from build123d import *

# Parameters (mm, degrees)
SKETCH1_W               = 44
SKETCH1_H               = 95
BOSS_EXTRUDE1_DEPTH     = 25
SKETCH2_W               = 38
SKETCH2_H               = 89
CUT_EXTRUDE1_DEPTH      = 22
CHAMFER1_SIZE           = 10
FILLET1_R               = 2
FILLET2_R               = 5
SKETCH3_W               = 14
SKETCH3_H               = 10
BOSS_EXTRUDE2_DEPTH     = 7
SKETCH5_W               = 14
SKETCH5_H               = 10
BOSS_EXTRUDE3_DEPTH     = 7
FILLET3_R               = 3
CUT_EXTRUDE2_DEPTH      = 62.010245041
CUT_EXTRUDE2_DEPTH_BACK = 62.010245041
SKETCH7_W               = 3
SKETCH7_H               = 6
SKETCH8_R               = 3
CUT_EXTRUDE3_DEPTH      = 10


with BuildPart() as part:
    # Sketch1 → Boss-Extrude1 (new body)
    with BuildSketch(Plane(origin=(0, 0, 0), x_dir=(1, 0, 0), z_dir=(0, 1, 0))):
        Rectangle(SKETCH1_W, SKETCH1_H)
    extrude(amount=BOSS_EXTRUDE1_DEPTH)

    # Sketch2 → Cut-Extrude1 (cut)
    with BuildSketch(Plane(origin=(0, 25, 0), x_dir=(1, 0, 0), z_dir=(0, 1, 0))):
        Rectangle(SKETCH2_W, SKETCH2_H)
    extrude(amount=-CUT_EXTRUDE1_DEPTH, mode=Mode.SUBTRACT)

    # Chamfer1
    chamfer1_edges = [part.edges().sort_by_distance(p)[0] for p in [
        (-19, 3, 0),
        (0, 3, -44.5),
        (19, 3, 0),
        (0, 3, 44.5),
        (0, 0, 47.5),
        (-22, 0, 0),
        (0, 0, -47.5),
        (22, 0, 0),
    ]]
    chamfer(chamfer1_edges, length=CHAMFER1_SIZE)

    # Fillet1
    fillet1_edges = [part.edges().sort_by_distance(p)[0] for p in [
        (-19, 19, -44.5),
        (19, 19, -44.5),
        (19, 19, 44.5),
        (-19, 19, 44.5),
    ]]
    fillet(fillet1_edges, radius=FILLET1_R)

    # Fillet2
    fillet2_edges = [part.edges().sort_by_distance(p)[0] for p in [
        (22, 17.5, 47.5),
        (-22, 17.5, 47.5),
        (-22, 17.5, -47.5),
        (22, 17.5, -47.5),
    ]]
    fillet(fillet2_edges, radius=FILLET2_R)

    # Sketch3 → Boss-Extrude2 (add)
    with BuildSketch(Plane(origin=(22, 0, 0), x_dir=(0, 0, -1), z_dir=(1, 0, 0))):
        with Locations((-32.5, 20)):
            Rectangle(SKETCH3_W, SKETCH3_H)
        with Locations((32.5, 20)):
            Rectangle(SKETCH3_W, SKETCH3_H)
    extrude(amount=BOSS_EXTRUDE2_DEPTH)

    # Sketch5 → Boss-Extrude3 (add)
    with BuildSketch(Plane.ZY.offset(22)):
        with Locations((32.5, 20)):
            Rectangle(SKETCH5_W, SKETCH5_H)
        with Locations((-32.5, 20)):
            Rectangle(SKETCH5_W, SKETCH5_H)
    extrude(amount=BOSS_EXTRUDE3_DEPTH)

    # Fillet3
    fillet3_edges = [part.edges().sort_by_distance(p)[0] for p in [
        (22, 20, 39.5),
        (22, 15, 32.5),
        (25.5, 15, 39.5),
        (22, 20, 25.5),
        (25.5, 15, 25.5),
        (29, 20, 39.5),
        (29, 15, 32.5),
        (29, 20, 25.5),
        (22, 20, -25.5),
        (22, 15, -32.5),
        (25.5, 15, -25.5),
        (22, 20, -39.5),
        (25.5, 15, -39.5),
        (29, 20, -25.5),
        (29, 15, -32.5),
        (29, 20, -39.5),
        (-22, 20, 39.5),
        (-25.5, 15, 39.5),
        (-22, 20, 25.5),
        (-22, 15, 32.5),
        (-25.5, 15, 25.5),
        (-29, 20, 39.5),
        (-29, 20, 25.5),
        (-29, 15, 32.5),
        (-22, 15, -32.5),
        (-25.5, 15, -39.5),
        (-22, 20, -25.5),
        (-25.5, 15, -25.5),
        (-22, 20, -39.5),
        (-29, 15, -32.5),
        (-29, 20, -25.5),
        (-29, 20, -39.5),
    ]]
    fillet(fillet3_edges, radius=FILLET3_R - 0.0001)  # a hair under: the kernel refuses the full size

    # Sketch7 → Cut-Extrude2 (cut, two sides: drawn at the far end of the back side and taken through both)
    with BuildSketch(Plane(origin=(0, 25, 0), x_dir=(1, 0, 0), z_dir=(0, 1, 0)).offset(-CUT_EXTRUDE2_DEPTH_BACK)):
        with Locations((-23.5, 32.5)):
            Rectangle(SKETCH7_W, SKETCH7_H)
        with Locations((23.5, 32.5)):
            Rectangle(SKETCH7_W, SKETCH7_H)
        with Locations((23.5, -32.5)):
            Rectangle(SKETCH7_W, SKETCH7_H)
        with Locations((-23.5, -32.5)):
            Rectangle(SKETCH7_W, SKETCH7_H)
    extrude(amount=CUT_EXTRUDE2_DEPTH + CUT_EXTRUDE2_DEPTH_BACK, mode=Mode.SUBTRACT)

    # Sketch8 → Cut-Extrude3 (cut)
    with BuildSketch(Plane.XY.offset(47.5)):
        with Locations((7, 25)):
            Circle(SKETCH8_R)
        with Locations((-7, 25)):
            Circle(SKETCH8_R)
    extrude(amount=-CUT_EXTRUDE3_DEPTH, mode=Mode.SUBTRACT)


solid = part.part
For this review, take the finished solid that the model builds, in its own axes (mm). A direction names the side the tool comes from. Coordinates: 2 decimals unless noted, no trailing zeros. Order: outer loops, then holes, each group sorted by start corner. A loop starts at its lowest first (then second) coordinate and runs counter-clockwise, first axis right, second up. Notation, with made-up numbers: (-33, 21.25) - (-17, 21.25) arc R25 ccw to (-17, 45.25) - close; hole circle Ø9 at (14, -1). An arc over 180 degrees is marked (long way). Use one line per item in the form item = value.
Q1. Consider section C-C (x = -7). Give the boundary of the cut face in (y, z), then the cut area to 3 significant figures.
Checked values:
outline = (0, -37.5) - (10, -47.5) - (25, -47.5) - (25, -44.5) - (13, -44.5) - (3, -34.5) - (3, 34.5) - (13, 44.5) - (22, 44.5) - (22, 47.5) - (10, 47.5) - (0, 37.5) - close
area = 408 mm2
Q2. Draft analysis for pull direction Z (two halves, no side actions). For faces 5 (the cylindrical face through (22.86, 14.1, -36.01)), 6 (the cylindrical face through (-28.1, 21.55, -26.36)), 7 (the cylindrical face through (20.5, 16.88, 46.07)), 8 (the cylindrical face through (28.14, 21.55, 26.4)), state which applies: +Z half, -Z half, draft (parallel to the pull), parting line (faces both ways), or undercut.
Checked values:
face_5 = draft
face_6 = undercut
face_7 = +Z half
face_8 = undercut
Q3. For P1, Ø0.9, axis at x = -23, y = 20, coming from the +Z side; P2, Ø5, axis at x = 11.5, z = -1, coming from the +Y side; P3, Ø0.8, axis at x = 25.5, y = 21, coming from the -Z side, all flat-tipped, find the tip position at first contact; note any pin that passes through.
Checked values:
P1 = 40.77
P2 = 8
P3 = -39.5
Q4. For probe 1 along X at (y, z) = (22.75, -35); probe 2 along Z at (x, y) = (-0.5, 23.75); probe 3 along Z at (x, y) = (22.5, 15.5), list the stretches that pass through material, from the lowest coordinate up. Write a range as from..to.
Checked values:
probe_1 = -29..-25, -22..-19, 19..22, 25..29
probe_2 = -47.5..-44.5, 44.5..47.5
probe_3 = -40.05..-35.5, -29.5..-24.95, 24.95..29.5, 35.5..40.05
Q5. For faces 1 (the flat face through (25, 20, -32)), 2 (the cylindrical face through (-25.51, 15.9, -38.64)), 3 (the cylindrical face through (18.43, 18.62, -43.9)), 4 (the cylindrical face through (22.86, 21.55, -24.6)), list the 3-axis set-ups (+Z, -Z, +X, -X, +Y, -Y) from which the entire face can be reached by the end or side of a thin tool; tool diameter is ignored.
Checked values:
face_1 = +Y, -Y
face_2 = -Z, -X, -Y
face_3 = +Y
face_4 = +X, +Y, -Y
Q6. Consider section B-B (x = -15). Give the boundary of the cut face in (y, z), then the cut area to 3 significant figures.
Checked values:
outline = (3, -40.5) - (10, -47.5) - (25, -47.5) - (25, -44.5) - (13, -44.5) - (9, -40.5) - (9, 40.5) - (13, 44.5) - (25, 44.5) - (25, 47.5) - (10, 47.5) - (3, 40.5) - close
area = 633 mm2
Q7. Consider section A-A (y = 7.25). Give the boundary of the cut face in (x, z).
Checked values:
outline = (-19.25, -44.75) - (19.25, -44.75) - (19.25, 44.75) - (-19.25, 44.75) - close; hole (-13.25, -38.75) - (13.25, -38.75) - (13.25, 38.75) - (-13.25, 38.75) - close
